Check sheet for the modelled part. Datum: model origin and axes. Units: mm. Give positions to 0.01 mm unless a question says otherwise; leave off trailing zeros. Loops run counter-clockwise (first coordinate to the right, second up) from the corner with the lowest first, then second, coordinate; pieces in that order, holes last. Notation, with made-up numbers: (74.5, 40) - (132.5, 40) arc R23 cw to (132.5, 73) - close; hole circle Ø10 at (-15, 5.25). An arc over 180 degrees is marked (long way). Use CSV: the item, a comma, the result in double quotes.
Autodesk Inventor part; units mm, degrees
ref_plane "YZ Plane" through (0, 0, 0) normal (1, 0, 0) x (0, 1, 0)
ref_plane "XZ Plane" through (0, 0, 0) normal (0, 1, 0) x (-1, 0, 0)
ref_plane "XY Plane" through (0, 0, 0) normal (0, 0, 1) x (1, 0, 0)
sketch "Эскиз1" plane through (0, 0, 0) normal (0, 1, 0) x (-1, 0, 0)
  circle A0 centre (0, 0) radius 65
  line L0 (0.182, -0.5) -> (62.998, -0.5)
  line L1 (62.998, 0.5) -> (1.3737, 0.5)
  line L2 (1.3737, 0.5) -> (48.5807, 40.1113)
  line L3 (47.9379, 40.8774) -> (-0.182, 0.5)
  line L4 (-0.182, 0.5) -> (-62.998, 0.5)
  line L5 (-62.998, -0.5) -> (-1.3737, -0.5)
  line L6 (-1.3737, -0.5) -> (-48.5807, -40.1113)
  line L7 (-47.9379, -40.8774) -> (0.182, -0.5)
  arc A1 (-62.998, -0.5) -> (-48.5807, -40.1113) centre (0, 0) ccw
  arc A2 (47.9379, 40.8774) -> (-62.998, 0.5) centre (0, 0) ccw
  arc A3 (-47.9379, -40.8774) -> (62.998, -0.5) centre (0, 0) ccw
  arc A4 (62.998, 0.5) -> (48.5807, 40.1113) centre (0, 0) ccw
  dimension "d1" = 130
extrude "Выдавливание1" add sketch "Эскиз1" along normal blind 5 contours A0 | L0 A3 L7 | L3 L4 A2
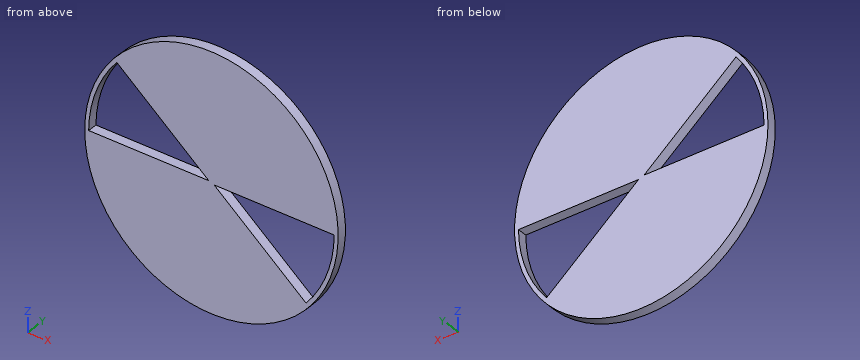
1. Sectioned sample at D-D, the plane z = -43.5. Record the boundary of the cut face in (x, y).
Completed:
outline,"(-48.3, 0) - (48.3, 0) - (48.3, 5) - (-48.3, 5) - close"
2. Go/stop test with flat-tipped pins: pin 1 Ø1.5 at (x, y) = (10.5, 2.5) entering from -Z; pin 2 Ø1.5 at (x, y) = (-45, 2.5) entering from +Z; pin 3 Ø1.5 at (y, z) = (1.5, -7.5) entering from -X. Record where each tip stops, or that it passes through.
Completed:
pin 1,"stops at z = -64.26"
pin 2,"stops at z = 47.61"
pin 3,"stops at x = -64.65"
3. Sectioned sample at B-B, the plane y = 2.65. Record the boundary of the cut face in (x, z).
Completed:
outline,"circle Ø130 at (0, 0); hole (-63, 0.5) - (-1.37, 0.5) - (-48.58, 40.11) arc R63 ccw to start; hole (1.37, -0.5) - (48.58, -40.11) arc R63 ccw to (63, -0.5) - close"
4. Sectioned sample at A-A, the plane x = -32. Record the boundary of the cut face in (y, z), and give its area (3 significant figures).
Completed:
outline,"(0, -56.58) - (5, -56.58) - (5, 0.5) - (0, 0.5) - close; (0, 26.2) - (5, 26.2) - (5, 56.58) - (0, 56.58) - close"
area,"437 mm²"
5. Sectioned sample at C-C, the plane z = 21. Record the boundary of the cut face in (x, y), and give its area (3 significant figures).
Completed:
outline,"(-61.51, 0) - (-59.4, 0) - (-59.4, 5) - (-61.51, 5) - close; (-25.8, 0) - (61.51, 0) - (61.51, 5) - (-25.8, 5) - close"
area,"447 mm²"
6. Scan lines: line 1 along Z through (x, y) = (-54, 1.3); line 2 along Z through (x, y) = (38, 1.05); line 3 along X through (y, z) = (3.2, -13). Record each from-to range of solid material in increasing order.
Completed:
line 1,"z = -36.18 to 0.5, 32.45 to 36.18"
line 2,"z = -52.74 to -31.23, -0.5 to 52.74"
line 3,"x = -63.69 to 16.27, 61.64 to 63.69"
